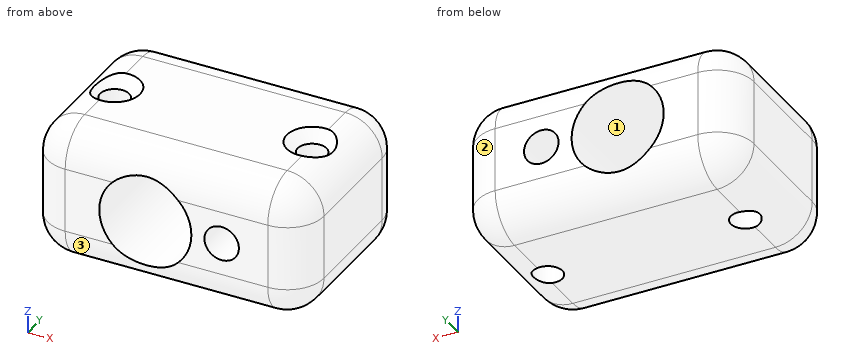
from build123d import *

# Parameters (mm, degrees)
F0_W           = 38.1
F0_H           = 19.05
F1_DEPTH       = 25.4
F2_D           = 12.7
F3_D           = 4.7625
F5_D           = 4
F5_CSINK_D     = 7
F5_CSINK_ANGLE = 90
F6_T1_DEPTH    = 27.94
F6_T3_DEPTH    = 15.24
F6_T5_DEPTH    = 8.89
F6_S9_W        = 5.08
F6_S9_H        = 5.08
F6_T10_DEPTH   = 5.08
F6_S15_W       = 5.08
F6_S15_H       = 5.08
F6_T16_DEPTH   = 5.08
F6_S21_W       = 5.08
F6_S21_H       = 5.08
F6_T22_DEPTH   = 5.08
F6_S27_W       = 5.08
F6_S27_H       = 5.08
F6_T28_DEPTH   = 5.08
F6_S33_W       = 5.08
F6_S33_H       = 5.08
F6_T34_DEPTH   = 5.08
F6_S39_W       = 5.08
F6_S39_H       = 5.08
F6_T40_DEPTH   = 5.08
F6_S45_W       = 5.08
F6_S45_H       = 5.08
F6_T46_DEPTH   = 5.08
F6_S51_W       = 5.08
F6_S51_H       = 5.08
F6_T52_DEPTH   = 5.08


# Not quite as in the source:
# - a fillet or chamfer that OpenCascade refuses, or shapes differently, is made with other operations: its cross-section is extruded or revolved along the edge and cut away or added


with BuildPart() as f1:
    # F0 (on Front) → F1 (new body)
    with BuildSketch(Plane.XZ):
        Rectangle(F0_W, F0_H)
    extrude(amount=F1_DEPTH)

    # F2 (through all)
    with Locations(Plane(origin=(0, 0, 0), x_dir=(1, 0, 0), z_dir=(0, 1, 0))):
        with Locations((-2.9169023037, 0)):
            Hole(F2_D / 2)

    # F3 (through all)
    with Locations(Plane(origin=(0, 0, 0), x_dir=(1, 0, 0), z_dir=(0, 1, 0))):
        with Locations((7.6106409542, 0)):
            Hole(F3_D / 2)

    # F5 (through all)
    with Locations(Plane.XY.offset(9.525)):
        with Locations((-13.6843686923, -12.9993055016), (13.5552566499, -12.9993055016)):
            CounterSinkHole(F5_D / 2, F5_CSINK_D / 2, counter_sink_angle=F5_CSINK_ANGLE)

    # F6: fillet of radius 5.08 on 12 edges, made by hand

    # F6_s2 → F6_t1 (cut)
    with BuildSketch(Plane.YZ.offset(-13.97)):
        with BuildLine():
            ThreePointArc((-5.08, 9.525), (-1.4878975516, 8.0371024484), (0, 4.445))
            Line((0, 4.445), (0, 9.525))
            Line((0, 9.525), (-5.08, 9.525))
        make_face()
        with BuildLine():
            ThreePointArc((-20.32, 9.525), (-23.9121024484, 8.0371024484), (-25.4, 4.445))
            Line((-25.4, 4.445), (-25.4, 9.525))
            Line((-25.4, 9.525), (-20.32, 9.525))
        make_face()
        with BuildLine():
            ThreePointArc((-20.32, -9.525), (-23.9121024484, -8.0371024484), (-25.4, -4.445))
            Line((-25.4, -4.445), (-25.4, -9.525))
            Line((-25.4, -9.525), (-20.32, -9.525))
        make_face()
        with BuildLine():
            ThreePointArc((-5.08, -9.525), (-1.4878975516, -8.0371024484), (0, -4.445))
            Line((0, -4.445), (0, -9.525))
            Line((0, -9.525), (-5.08, -9.525))
        make_face()
    extrude(amount=F6_T1_DEPTH, mode=Mode.SUBTRACT)

    # F6_s4 → F6_t3 (cut)
    with BuildSketch(Plane.XZ.offset(5.08)):
        with BuildLine():
            ThreePointArc((13.97, -9.525), (17.5621024484, -8.0371024484), (19.05, -4.445))
            Line((19.05, -4.445), (19.05, -9.525))
            Line((19.05, -9.525), (13.97, -9.525))
        make_face()
        with BuildLine():
            ThreePointArc((13.97, 9.525), (17.5621024484, 8.0371024484), (19.05, 4.445))
            Line((19.05, 4.445), (19.05, 9.525))
            Line((19.05, 9.525), (13.97, 9.525))
        make_face()
        with BuildLine():
            ThreePointArc((-19.05, 4.445), (-17.5621024484, 8.0371024484), (-13.97, 9.525))
            Line((-13.97, 9.525), (-19.05, 9.525))
            Line((-19.05, 9.525), (-19.05, 4.445))
        make_face()
        with BuildLine():
            ThreePointArc((-19.05, -4.445), (-17.5621024484, -8.0371024484), (-13.97, -9.525))
            Line((-13.97, -9.525), (-19.05, -9.525))
            Line((-19.05, -9.525), (-19.05, -4.445))
        make_face()
    extrude(amount=F6_T3_DEPTH, mode=Mode.SUBTRACT)

    # F6_s6 → F6_t5 (cut)
    with BuildSketch(Plane.XY.offset(-4.445)):
        with BuildLine():
            ThreePointArc((13.97, 0), (17.5621024484, -1.4878975516), (19.05, -5.08))
            Line((19.05, -5.08), (19.05, 0))
            Line((19.05, 0), (13.97, 0))
        make_face()
        with BuildLine():
            ThreePointArc((13.97, -25.4), (17.5621024484, -23.9121024484), (19.05, -20.32))
            Line((19.05, -20.32), (19.05, -25.4))
            Line((19.05, -25.4), (13.97, -25.4))
        make_face()
        with BuildLine():
            ThreePointArc((-19.05, -5.08), (-17.5621024484, -1.4878975516), (-13.97, 0))
            Line((-13.97, 0), (-19.05, 0))
            Line((-19.05, 0), (-19.05, -5.08))
        make_face()
        with BuildLine():
            ThreePointArc((-19.05, -20.32), (-17.5621024484, -23.9121024484), (-13.97, -25.4))
            Line((-13.97, -25.4), (-19.05, -25.4))
            Line((-19.05, -25.4), (-19.05, -20.32))
        make_face()
    extrude(amount=F6_T5_DEPTH, mode=Mode.SUBTRACT)


with BuildPart() as f6_tool8:
    # F6_s9 → F6_t10 (new body)
    with BuildSketch(Plane.XY.offset(4.445)):
        with Locations((16.51, -2.54)):
            Rectangle(F6_S9_W, F6_S9_H)
    extrude(amount=F6_T10_DEPTH)

    # F6_s11 → F6_t12 (revolve, cut)
    with BuildSketch(Plane(origin=(13.97, -5.08, 4.445), x_dir=(-0.7071067812, -0.7071067812, 0), z_dir=(-0.7071067812, 0.7071067812, 0))):
        with BuildLine():
            ThreePointArc((0, -5.08), (5.08, 0), (0, 5.08))
            Line((0, 5.08), (0, -5.08))
        make_face()
    revolve(axis=Axis((13.97, -5.08, 4.445), (0, 0, 1)), mode=Mode.SUBTRACT)


with BuildPart() as f1_1:
    add(f1.part)

    # F6_t7: cut F6_tool8
    add(f6_tool8.part, mode=Mode.SUBTRACT)


with BuildPart() as f6_tool14:
    # F6_s15 → F6_t16 (new body)
    with BuildSketch(Plane.YZ.offset(-13.97)):
        with Locations((-2.54, 6.985)):
            Rectangle(F6_S15_W, F6_S15_H)
    extrude(amount=-F6_T16_DEPTH)

    # F6_s17 → F6_t18 (revolve, cut)
    with BuildSketch(Plane(origin=(-13.97, -5.08, 4.445), x_dir=(0, -0.7071067812, -0.7071067812), z_dir=(0, 0.7071067812, -0.7071067812))):
        with BuildLine():
            ThreePointArc((0, -5.08), (5.08, 0), (0, 5.08))
            Line((0, 5.08), (0, -5.08))
        make_face()
    revolve(axis=Axis((-13.97, -5.08, 4.445), (-1, 0, 0)), mode=Mode.SUBTRACT)


with BuildPart() as f1_2:
    add(f1_1.part)

    # F6_t13: cut F6_tool14
    add(f6_tool14.part, mode=Mode.SUBTRACT)


with BuildPart() as f6_tool20:
    # F6_s21 → F6_t22 (new body)
    with BuildSketch(Plane.XY.offset(4.445)):
        with Locations((16.51, -22.86)):
            Rectangle(F6_S21_W, F6_S21_H)
    extrude(amount=F6_T22_DEPTH)

    # F6_s23 → F6_t24 (revolve, cut)
    with BuildSketch(Plane(origin=(13.97, -20.32, 4.445), x_dir=(-0.7071067812, 0.7071067812, 0), z_dir=(0.7071067812, 0.7071067812, 0))):
        with BuildLine():
            ThreePointArc((0, -5.08), (5.08, 0), (0, 5.08))
            Line((0, 5.08), (0, -5.08))
        make_face()
    revolve(axis=Axis((13.97, -20.32, 4.445), (0, 0, 1)), mode=Mode.SUBTRACT)


with BuildPart() as f1_3:
    add(f1_2.part)

    # F6_t19: cut F6_tool20
    add(f6_tool20.part, mode=Mode.SUBTRACT)


with BuildPart() as f6_tool26:
    # F6_s27 → F6_t28 (new body)
    with BuildSketch(Plane.YZ.offset(-13.97)):
        with Locations((-22.86, 6.985)):
            Rectangle(F6_S27_W, F6_S27_H)
    extrude(amount=-F6_T28_DEPTH)

    # F6_s29 → F6_t30 (revolve, cut)
    with BuildSketch(Plane(origin=(-13.97, -20.32, 4.445), x_dir=(0, 0.7071067812, -0.7071067812), z_dir=(0, 0.7071067812, 0.7071067812))):
        with BuildLine():
            ThreePointArc((0, -5.08), (5.08, 0), (0, 5.08))
            Line((0, 5.08), (0, -5.08))
        make_face()
    revolve(axis=Axis((-13.97, -20.32, 4.445), (-1, 0, 0)), mode=Mode.SUBTRACT)


with BuildPart() as f1_4:
    add(f1_3.part)

    # F6_t25: cut F6_tool26
    add(f6_tool26.part, mode=Mode.SUBTRACT)


with BuildPart() as f6_tool32:
    # F6_s33 → F6_t34 (new body)
    with BuildSketch(Plane.YZ.offset(-13.97)):
        with Locations((-22.86, -6.985)):
            Rectangle(F6_S33_W, F6_S33_H)
    extrude(amount=-F6_T34_DEPTH)

    # F6_s35 → F6_t36 (revolve, cut)
    with BuildSketch(Plane(origin=(-13.97, -20.32, -4.445), x_dir=(0, 0.7071067812, 0.7071067812), z_dir=(0, -0.7071067812, 0.7071067812))):
        with BuildLine():
            ThreePointArc((0, -5.08), (5.08, 0), (0, 5.08))
            Line((0, 5.08), (0, -5.08))
        make_face()
    revolve(axis=Axis((-13.97, -20.32, -4.445), (-1, 0, 0)), mode=Mode.SUBTRACT)


with BuildPart() as f1_5:
    add(f1_4.part)

    # F6_t31: cut F6_tool32
    add(f6_tool32.part, mode=Mode.SUBTRACT)


with BuildPart() as f6_tool38:
    # F6_s39 → F6_t40 (new body)
    with BuildSketch(Plane.XY.offset(-4.445)):
        with Locations((16.51, -22.86)):
            Rectangle(F6_S39_W, F6_S39_H)
    extrude(amount=-F6_T40_DEPTH)

    # F6_s41 → F6_t42 (revolve, cut)
    with BuildSketch(Plane(origin=(13.97, -20.32, -4.445), x_dir=(-0.7071067812, 0.7071067812, 0), z_dir=(-0.7071067812, -0.7071067812, 0))):
        with BuildLine():
            ThreePointArc((0, -5.08), (5.08, 0), (0, 5.08))
            Line((0, 5.08), (0, -5.08))
        make_face()
    revolve(axis=Axis((13.97, -20.32, -4.445), (0, 0, -1)), mode=Mode.SUBTRACT)


with BuildPart() as f1_6:
    add(f1_5.part)

    # F6_t37: cut F6_tool38
    add(f6_tool38.part, mode=Mode.SUBTRACT)


with BuildPart() as f6_tool44:
    # F6_s45 → F6_t46 (new body)
    with BuildSketch(Plane.YZ.offset(-13.97)):
        with Locations((-2.54, -6.985)):
            Rectangle(F6_S45_W, F6_S45_H)
    extrude(amount=-F6_T46_DEPTH)

    # F6_s47 → F6_t48 (revolve, cut)
    with BuildSketch(Plane(origin=(-13.97, -5.08, -4.445), x_dir=(0, -0.7071067812, 0.7071067812), z_dir=(0, -0.7071067812, -0.7071067812))):
        with BuildLine():
            ThreePointArc((0, -5.08), (5.08, 0), (0, 5.08))
            Line((0, 5.08), (0, -5.08))
        make_face()
    revolve(axis=Axis((-13.97, -5.08, -4.445), (-1, 0, 0)), mode=Mode.SUBTRACT)


with BuildPart() as f1_7:
    add(f1_6.part)

    # F6_t43: cut F6_tool44
    add(f6_tool44.part, mode=Mode.SUBTRACT)


with BuildPart() as f6_tool50:
    # F6_s51 → F6_t52 (new body)
    with BuildSketch(Plane.XY.offset(-4.445)):
        with Locations((16.51, -2.54)):
            Rectangle(F6_S51_W, F6_S51_H)
    extrude(amount=-F6_T52_DEPTH)

    # F6_s53 → F6_t54 (revolve, cut)
    with BuildSketch(Plane(origin=(13.97, -5.08, -4.445), x_dir=(-0.7071067812, -0.7071067812, 0), z_dir=(0.7071067812, -0.7071067812, 0))):
        with BuildLine():
            ThreePointArc((0, -5.08), (5.08, 0), (0, 5.08))
            Line((0, 5.08), (0, -5.08))
        make_face()
    revolve(axis=Axis((13.97, -5.08, -4.445), (0, 0, -1)), mode=Mode.SUBTRACT)


with BuildPart() as f1_8:
    add(f1_7.part)

    # F6_t49: cut F6_tool50
    add(f6_tool50.part, mode=Mode.SUBTRACT)


solid = f1_8.part
Input: part model. Units: mm. Frame: model coordinates. Face numbers are marked on the shaded views. Give positions to 0.01 mm unless a question says otherwise; leave off trailing zeros. Order: outer loops, then holes, each group sorted by start corner. A loop starts at its lowest first (then second) coordinate and runs counter-clockwise, first axis right, second up. Notation, with made-up numbers: (22, 85) - (48, 85) arc R27 cw to (48, 119) - close; hole circle Ø3 at (0.5, 70.5). An arc over 180 degrees is marked (long way). Write each question's results on one line, items separated by ' | '.
Item 1: Section B-B (y = -17.25). Give the number of separate pieces and of enclosed holes in the cut face, and give its area (3 significant figures).
A:
separate pieces: 1 | enclosed holes: 2 | area: 559 mm^2
Item 2: Draft query along X for the marked faces 1, 2 and 3. Return one class per face: released by +X, released by -X, zero draft, split by the parting line, or undercut.
A:
face 1: undercut | face 2: released by +X | face 3: zero draft
Item 3: Section D-D (z = -3.75). Return loops of the section in (x, y).
A:
outline: (-19.05, -20.32) arc R5.08 ccw to (-13.97, -25.4) - (-8.04, -25.4) - (-8.04, 0) - (-13.97, 0) arc R5.08 ccw to (-19.05, -5.08) - close; (2.21, -25.4) - (13.97, -25.4) arc R5.08 ccw to (19.05, -20.32) - (19.05, -5.08) arc R5.08 ccw to (13.97, 0) - (2.21, 0) - close; hole circle Ø4 at (-13.68, -13); hole circle Ø4 at (13.56, -13)
Item 4: Material intervals for line 1 along X through (y, z) = (-17, -2); line 2 along X through (y, z) = (-17.25, 1); line 3 along X through (y, z) = (-13.5, -5), sorted ascending.
A:
line 1: x = -19.05 to -8.94, 3.11 to 6.32, 8.9 to 19.05 | line 2: x = -19.05 to -9.19, 3.35 to 5.45, 9.77 to 19.05 | line 3: x = -19.02 to -15.62, -11.75 to -6.83, 1 to 11.62, 15.49 to 19.02
Item 5: Section C-C (x = 1). Return loops of the section in (y, z) (3 decimals).
A:
outline: (-25.37, -4.998) arc R5.08 ccw to (-20.32, -9.525) - (-5.08, -9.525) arc R5.08 ccw to (-0.03, -4.998) - close; (-25.37, 4.998) - (-0.03, 4.998) arc R5.08 ccw to (-5.08, 9.525) - (-20.32, 9.525) arc R5.08 ccw to start
Item 6: Section A-A (z = 0.5). Return loops of the section in (x, y).
A:
outline: (-19.05, -20.32) arc R5.08 ccw to (-13.97, -25.4) - (-9.25, -25.4) - (-9.25, 0) - (-13.97, 0) arc R5.08 ccw to (-19.05, -5.08) - close; (3.41, -25.4) - (5.28, -25.4) - (5.28, 0) - (3.41, 0) - close; (9.94, -25.4) - (13.97, -25.4) arc R5.08 ccw to (19.05, -20.32) - (19.05, -5.08) arc R5.08 ccw to (13.97, 0) - (9.94, 0) - close; hole circle Ø4 at (-13.68, -13); hole circle Ø4 at (13.56, -13)
